The figure shows three views and two pictorial views of one solid part (mm, origin at its lowest corner). Answer the questions. Give positions to 0.01 mm unless a question says otherwise; leave off trailing zeros. Order: outer loops, then holes, each group sorted by start corner. A loop starts at its lowest first (then second) coordinate and runs counter-clockwise, first axis right, second up. Notation, with made-up numbers: (77, -27.5) - (102, -27.5) arc R10 ccw to (102, -19.5) - close; hole circle Ø1 at (19, 63). An arc over 180 degrees is marked (long way). Use a Markdown table: item, result. Add a question column.
1. A cutting plane is placed at A-A on z = 14. Determine the outline of the cut face in (x, y).
2. Consider L1, parallel to Y at x = 7.5, z = 6.25; L2, parallel to X at y = 5.5, z = 8.5; L3, parallel to X at y = 9.75, z = 3 (1 decimal). Determine where each line is inside the solid, lowest interval first.
3. A cutting plane is placed at B-B on x = 1.5. Determine the outline of the cut face in (y, z).
4. Flat-ended cylindrical pins translate along their axes: P1, Ø2, axis at y = 2, z = 20, coming from the -X side; P2, Ø1.5, axis at y = 9, z = 46, coming from the -X side; P3, Ø2, axis at y = 5, z = 47, coming from the +X side. Find the tip coordinate at first contact, or state that the pin passes through.
5. A cutting plane is placed at D-D on z = 39.5. Determine the outline of the cut face in (x, y), and give its area (3 significant figures).
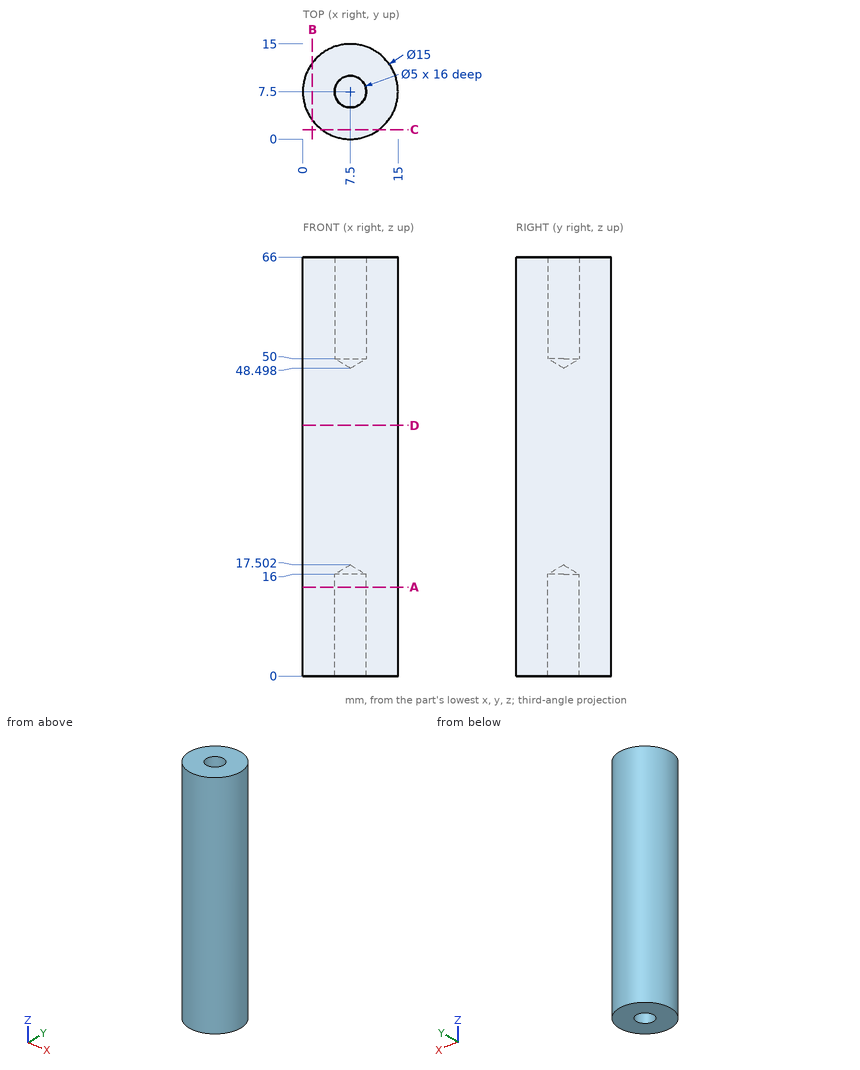
Output values:
| question | item | result |
|---|---|---|
| 1 | outline | circle Ø15 at (7.5, 7.5); hole circle Ø5 at (7.5, 7.5) |
| 2 | L1 | 0 to 5, 10 to 15 |
| 2 | L2 | 0.27 to 6, 9 to 14.73 |
| 2 | L3 | 0.3 to 6.4, 8.6 to 14.7 |
| 3 | outline | (3, 0) - (12, 0) - (12, 66) - (3, 66) - close |
| 4 | P1 | x = 1.5 |
| 4 | P2 | x = 0.04 |
| 4 | P3 | x = 14.85 |
| 5 | outline | circle Ø15 at (7.5, 7.5) |
| 5 | area | 177 mm² |
